from build123d import *

# Parameters (mm, degrees)
F0_R     = 51.9492240189
F1_DEPTH = 25.4
F2_DEPTH = 94.488
F5_D     = 14.986
F6_R     = 5.08


with BuildPart() as f1:
    # F0 (on Front) → F1 (new body)
    with BuildSketch(Plane.XZ):
        Circle(F0_R)
    extrude(amount=F1_DEPTH)

    # F2 (add): a face of the model
    f2_faces = [f1.faces().sort_by_distance(p)[0] for p in [
        (0, -25.4, 0),
    ]]
    extrude(f2_faces, amount=F2_DEPTH)

    # F5 (through all)
    with Locations(Plane.XZ.offset(119.888)):
        with Locations((0, 0)):
            Hole(F5_D / 2)

    # F6
    f6_edges = [f1.edges().sort_by_distance(p)[0] for p in [
        (-51.949224, -119.888, 0),
        (-51.949224, 0, 0),
        (-7.493, 0, 0),
        (-7.493, -119.888, 0),
    ]]
    fillet(f6_edges, radius=F6_R)


solid = f1.part
The model under review builds one solid part; all positions refer to its coordinate system, in mm. Coordinates: 2 decimals unless noted, no trailing zeros. Write each loop counter-clockwise with the first axis right and the second up, starting at its lowest first coordinate (ties: lowest second). Pieces come first, ordered by that corner, then holes. Notation, with made-up numbers: M -23.5,67 L 13.5,67 A25 cw 13.5,95 Z; hole C 54.25,82 d2. An arc over 180 degrees is marked long. Put each result on its own line as item: value.
1) Draft analysis for pull direction X (two halves, no side actions). For faces 1 (the cylindrical face through (0.98, -59.18, 7.43)), 2 (the cylindrical face through (49.55, -59.18, 15.6)), 3 (the flat face through (10, 0, -10)), state which applies: released by +X, released by -X, zero draft, split by the parting line, or undercut.
Computed:
face 1: undercut
face 2: split by the parting line
face 3: zero draft
2) Add section C-C on y = -94. Give the boundary of the cut face in (x, z), then the cut area to 3 significant figures.
Computed:
outline: C 0,0 d103.9; hole C 0,0 d14.99
area: 8,300 mm2
3) Add section B-B on x = 0. Give the boundary of the cut face in (y, z), then the cut area to 3 significant figures.
Computed:
outline: M -119.89,-46.87 A5.08 ccw -114.81,-51.95 L -5.08,-51.95 A5.08 ccw 0,-46.87 L 0,-12.57 A5.08 ccw -5.08,-7.49 L -114.81,-7.49 A5.08 ccw -119.89,-12.57 Z; M -119.89,12.57 A5.08 ccw -114.81,7.49 L -5.08,7.49 A5.08 ccw 0,12.57 L 0,46.87 A5.08 ccw -5.08,51.95 L -114.81,51.95 A5.08 ccw -119.89,46.87 Z
area: 10,600 mm2
4) Clearance check with flat-ended pins moving along their axes: pin 1 Ø1 at (x, y) = (22, -42) entering from -Z; pin 2 Ø6 at (x, y) = (-21, -80) entering from +Z; pin 3 Ø1.5 at (x, y) = (22, -46.5) entering from +Z. State where each tip first meets the part, or that it passes through.
Computed:
pin 1: stops at z = -47.29
pin 2: stops at z = 48.73
pin 3: stops at z = 47.4
5) Wall thickness on probe 1 along Z at (x, y) = (0, -81); probe 2 along X at (y, z) = (-15, 6); probe 3 along X at (y, z) = (-63, 5): over which ranges is each line inside the solid? List them lowest first. Write a range as [from, to].
Computed:
probe 1: z = [-51.95, -7.49], [7.49, 51.95]
probe 2: x = [-51.6, -4.49], [4.49, 51.6]
probe 3: x = [-51.71, -5.58], [5.58, 51.71]
6) Add section A-A on z = 0. Give the boundary of the cut face in (x, y), then the cut area to 3 significant figures.
Computed:
outline: M -51.95,-114.81 A5.08 ccw -46.87,-119.89 L -12.57,-119.89 A5.08 ccw -7.49,-114.81 L -7.49,-5.08 A5.08 ccw -12.57,0 L -46.87,0 A5.08 ccw -51.95,-5.08 Z; M 7.49,-114.81 A5.08 ccw 12.57,-119.89 L 46.87,-119.89 A5.08 ccw 51.95,-114.81 L 51.95,-5.08 A5.08 ccw 46.87,0 L 12.57,0 A5.08 ccw 7.49,-5.08 Z
area: 10,600 mm2
